from build123d import *

# Parameters (mm, degrees)
F0_W     = 100
F0_H     = 150
F1_DEPTH = 40
F3_D     = 20
F4_SIZE  = 5
F5_R     = 5


with BuildPart() as f1:
    # F0 (on Front) → F1 (new body, symmetric)
    with BuildSketch(Plane.XZ):
        Rectangle(F0_W, F0_H)
    extrude(amount=F1_DEPTH, both=True)

    # F3 (through all)
    with Locations(Plane.XY.offset(75)):
        with Locations((-30, 0)):
            Hole(F3_D / 2)

    # F4
    f4_edges = [f1.edges().sort_by_distance(p)[0] for p in [
        (-50, 0, 75),
    ]]
    chamfer(f4_edges, length=F4_SIZE)

    # F5
    f5_edges = [f1.edges().sort_by_distance(p)[0] for p in [
        (50, 0, 75),
    ]]
    fillet(f5_edges, radius=F5_R)


solid = f1.part
Work out the finished part from the listing and answer in its coordinate system (mm). Coordinates: 2 decimals unless noted, no trailing zeros. Write each loop counter-clockwise with the first axis right and the second up, starting at its lowest first coordinate (ties: lowest second). Pieces come first, ordered by that corner, then holes. Notation, with made-up numbers: M 46,-32 L 51,-32 A16 cw 51,-25 Z; hole C 29.25,75 d7. An arc over 180 degrees is marked long. Write item = value, one per line.
1. The part is cut by section C-C (z = 43.5). Determine the outline of the cut face in (x, y), then the cut area to 3 significant figures.
Solution:
outline = M -50,-40 L 50,-40 L 50,40 L -50,40 Z; hole C -30,0 d20
area = 7,690 mm2
2. Determine the mould class of faces 1 (the face through (-1, 40, 1)), 2 (the face through (-39.54, 3, -1.05)), 3 (the face through (48, 1, 74)) for opening direction Y: released by +Y, released by -Y, zero draft, split by the parting line, or undercut.
Solution:
face_1 = released by +Y
face_2 = undercut
face_3 = zero draft
3. The part is cut by section A-A (y = 0). Determine the outline of the cut face in (x, z), then the cut area to 3 significant figures.
Solution:
outline = M -50,-75 L -40,-75 L -40,75 L -45,75 L -50,70 Z; M -20,-75 L 50,-75 L 50,70 A5 ccw 45,75 L -20,75 Z
area = 12,000 mm2
4. Straight lines are drawn through the part: line 1 (Y direction, x = -30, z = -38); line 2 (X direction, y = -6, z = 56); line 3 (Y direction, x = -25.5, z = 30). For each, find the intervals that lie inside material, in ascending order. Write a range as from..to.
Solution:
line_1 = -40..-10, 10..40
line_2 = -50..-38, -22..50
line_3 = -40..-8.93, 8.93..40
5. The part is cut by section B-B (x = -30). Determine the outline of the cut face in (y, z).
Solution:
outline = M -40,-75 L -10,-75 L -10,75 L -40,75 Z; M 10,-75 L 40,-75 L 40,75 L 10,75 Z
